Work out the finished part from the listing and answer in its coordinate system (mm). A direction names the side the tool comes from. Give positions to 0.01 mm unless a question says otherwise; leave off trailing zeros. Order: outer loops, then holes, each group sorted by start corner. A loop starts at its lowest first (then second) coordinate and runs counter-clockwise, first axis right, second up. Notation, with made-up numbers: M 30,23 L 83,23 A24 ccw 83,62 Z; hole C 24,-13 d7. An arc over 180 degrees is marked long. One line per item, written item: value.
from build123d import *

# Parameters (mm, degrees)
BOSS_EXTRUDE1_DEPTH  = 5
SKETCH2_R            = 5
CUT_EXTRUDE1_DEPTH   = 5
SKETCH4_W            = 28.341926147
SKETCH4_H            = 5
BOSS_EXTRUDE2_DEPTH  = 5
SKETCH5_W            = 28.341926147
SKETCH5_H            = 5
BOSS_EXTRUDE3_DEPTH  = 31.9
SKETCH6_W            = 20
SKETCH6_H            = 5
CUT_EXTRUDE3_DEPTH   = 5
SKETCH8_W            = 4.170963073
SKETCH8_H            = 5
SKETCH8_W_2          = 4.170963074
BOSS_EXTRUDE8_DEPTH  = 10
SKETCH15_W           = 20
SKETCH15_H           = 5
BOSS_EXTRUDE9_DEPTH  = 5
SKETCH18_W           = 28.341926147
SKETCH18_H           = 5
BOSS_EXTRUDE11_DEPTH = 12.11
SKETCH19_R           = 1
CUT_EXTRUDE6_DEPTH   = 12.11
BOSS_EXTRUDE12_START = 5
SKETCH20_R           = 10
BOSS_EXTRUDE12_DEPTH = 5


with BuildPart() as part:
    # Model → Boss-Extrude1 (new body)
    with BuildSketch(Plane.XY):
        with BuildLine():
            Line((25.203972036, 18.418809181), (53.545898183, 18.418809181))
            ThreePointArc((53.545898183, 18.418809181), (56.325296764, 25.33096224), (62.273132312, 29.817182103))
            ThreePointArc((62.273132312, 29.817182103), (70.250885109, 48.157178295), (51.910888918, 56.134931092))
            ThreePointArc((51.910888918, 56.134931092), (32.934484586, 41.258497646), (25.203972036, 18.418809181))
        make_face()
    extrude(amount=BOSS_EXTRUDE1_DEPTH)

    # Sketch2 → Cut-Extrude1 (cut)
    with BuildSketch(Plane.XY.offset(5)):
        with Locations((57.092010615, 42.976056598)):
            Circle(SKETCH2_R)
    extrude(amount=-CUT_EXTRUDE1_DEPTH, mode=Mode.SUBTRACT)

    # Sketch4 → Boss-Extrude2 (add)
    with BuildSketch(Plane.XZ.offset(-18.418809181)):
        with Locations((39.37493511, 2.5)):
            Rectangle(SKETCH4_W, SKETCH4_H)
    extrude(amount=BOSS_EXTRUDE2_DEPTH)

    # Sketch5 → Boss-Extrude3 (add)
    with BuildSketch(Plane(origin=(0, 0, 0), x_dir=(-1, 0, 0), z_dir=(0, 0, -1))):
        with Locations((-39.37493511, 15.918809181)):
            Rectangle(SKETCH5_W, SKETCH5_H)
    extrude(amount=BOSS_EXTRUDE3_DEPTH)

    # Sketch6 → Cut-Extrude3 (cut)
    with BuildSketch(Plane(origin=(0, 18.418809181, 0), x_dir=(1, 0, 0), z_dir=(0, 1, 0))):
        with Locations((39.37493511, 29.4)):
            Rectangle(SKETCH6_W, SKETCH6_H)
    extrude(amount=-CUT_EXTRUDE3_DEPTH, mode=Mode.SUBTRACT)

    # Sketch8 → Boss-Extrude8 (add)
    with BuildSketch(Plane(origin=(0, 0, -31.9), x_dir=(-1, 0, 0), z_dir=(0, 0, -1))):
        with Locations((-51.460416647, 15.918809181)):
            Rectangle(SKETCH8_W, SKETCH8_H)
        with Locations((-27.289453573, 15.918809181)):
            Rectangle(SKETCH8_W_2, SKETCH8_H)
    extrude(amount=BOSS_EXTRUDE8_DEPTH)

    # Sketch15 → Boss-Extrude9 (add)
    with BuildSketch(Plane(origin=(0, 0, -26.9), x_dir=(-1, 0, 0), z_dir=(0, 0, -1))):
        with Locations((-39.37493511, 15.918809181)):
            Rectangle(SKETCH15_W, SKETCH15_H)
    extrude(amount=BOSS_EXTRUDE9_DEPTH)

    # Sketch18 → Boss-Extrude11 (add)
    with BuildSketch(Plane(origin=(0, 0, -41.9), x_dir=(-1, 0, 0), z_dir=(0, 0, -1))):
        with Locations((-39.37493511, 15.918809181)):
            Rectangle(SKETCH18_W, SKETCH18_H)
    extrude(amount=BOSS_EXTRUDE11_DEPTH)

    # Sketch19 → Cut-Extrude6 (cut)
    with BuildSketch(Plane(origin=(0, 18.418809181, 0), x_dir=(1, 0, 0), z_dir=(0, 1, 0))):
        with Locations(Location((34.37493511, 22, 0), (0, 0, 270))):
            Circle(SKETCH19_R)
        with Locations(Location((44.37493511, 22, 0), (0, 0, 270))):
            Circle(SKETCH19_R)
        with Locations(Location((34.37493511, 15, 0), (0, 0, 270))):
            Circle(SKETCH19_R)
        with Locations(Location((44.37493511, 15, 0), (0, 0, 270))):
            Circle(SKETCH19_R)
    extrude(amount=-CUT_EXTRUDE6_DEPTH, mode=Mode.SUBTRACT)

    # Sketch20 → Boss-Extrude12 (add)
    with BuildSketch(Plane(origin=(0, 0, -54.01), x_dir=(-1, 0, 0), z_dir=(0, 0, -1)).offset(BOSS_EXTRUDE12_START)):
        with BuildLine():
            Line((-53.545898183, 18.418809181), (-53.545898183, 13.418809181))
            Line((-53.545898183, 13.418809181), (-25.203972036, 13.418809181))
            Line((-25.203972036, 13.418809181), (-25.203972036, 18.418809181))
            ThreePointArc((-25.203972036, 18.418809181), (-32.934484586, 41.258497646), (-51.910888918, 56.134931092))
            ThreePointArc((-51.910888918, 56.134931092), (-70.250885109, 48.157178295), (-62.273132312, 29.817182103))
            ThreePointArc((-62.273132312, 29.817182103), (-56.325296764, 25.33096224), (-53.545898183, 18.418809181))
        make_face()
        with Locations((-57.092010615, 42.976056598)):
            Circle(SKETCH20_R, mode=Mode.SUBTRACT)
    extrude(amount=-BOSS_EXTRUDE12_DEPTH)


solid = part.part
(1) Section C-C, the plane y = 40 is taken. Give the vertices of the cut face in (x, z).
Findings:
outline: M 32.08,-59.01 L 47.55,-59.01 L 47.55,-54.01 L 32.08,-54.01 Z; M 32.08,0 L 53.07,0 L 53.07,5 L 32.08,5 Z; M 61.11,0 L 70.92,0 L 70.92,5 L 61.11,5 Z; M 66.64,-59.01 L 70.92,-59.01 L 70.92,-54.01 L 66.64,-54.01 Z
(2) Which of the six approach directions +Z, -Z, +X, -X, +Y, -Y give full straight-line access (tool end or side, diameter ignored) to faces 4 (the flat face through (48, 38, 0)), 5 (the cylindrical face through (52.478, 34.104, -56.545)), 6 (the flat face through (40, 13.419, -27)), 7 (the flat face through (29.375, 16, -37)), 8 (the cylindrical face through (56.261, 25.247, 2.465))?
Findings:
face 4: +X, -X, +Y
face 5: -Z
face 6: +Z, -Z, +X, -X, -Y
face 7: +Y, -Y
face 8: +Z, -Z, +X, -Y
(3) Section A-A, the plane z = -34 is taken. Give the vertices of the cut face in (x, y).
Findings:
outline: M 25.2,13.42 L 29.37,13.42 L 29.37,18.42 L 25.2,18.42 Z; M 49.37,13.42 L 53.55,13.42 L 53.55,18.42 L 49.37,18.42 Z
(4) Section D-D, the plane x = 61 is taken. Give the vertices of the cut face in (y, z).
Findings:
outline: M 29.24,-59.01 L 33.77,-59.01 L 33.77,-54.01 L 29.24,-54.01 Z; M 29.24,0 L 39.86,0 L 39.86,5 L 29.24,5 Z; M 46.09,0 L 56.57,0 L 56.57,5 L 46.09,5 Z; M 52.18,-59.01 L 56.57,-59.01 L 56.57,-54.01 L 52.18,-54.01 Z
(5) Section B-B, the plane z = -22 is taken. Give the vertices of the cut face in (x, y).
Findings:
outline: M 25.2,13.42 L 33.37,13.42 L 33.37,18.42 L 25.2,18.42 Z; M 35.37,13.42 L 43.37,13.42 L 43.37,18.42 L 35.37,18.42 Z; M 45.37,13.42 L 53.55,13.42 L 53.55,18.42 L 45.37,18.42 Z
(6) Determine the mould class of faces 1 (the cylindrical face through (35.218, 15.954, -14.462)), 2 (the cylindrical face through (70.36, 47.87, 2.46)), 3 (the flat face through (43, 31, -59.01)) for opening direction Z: pulls with the +Z half, pulls with the -Z half, needs draft (parallel to the pull), parting line crosses it, or undercut.
Findings:
face 1: undercut
face 2: needs draft
face 3: pulls with the -Z half
(7) Find the intervals of material crossed by probe 1 along X at (y, z) = (16.25, -22); probe 2 along Z at (x, y) = (44.5, 27.5); probe 3 along Z at (x, y) = (59, 49), in increasing order. Write a range as from..to.
Findings:
probe 1: x = 25.2..33.37, 35.37..43.37, 45.37..53.55
probe 2: z = -59.01..-54.01, 0..5
probe 3: z = 0..5
(8) Given P1, Ø1.5, axis at y = 16.5, z = -23.5, coming from the +X side; P2, Ø8.5, axis at x = 39, z = -31, coming from the +Y side; P3, Ø1.2, axis at x = 34.37, z = -15, coming from the -Y side, each flat-ended and moving along its own axis, determine where each tip first touches the part or whether it passes through.
Findings:
P1: stops at x = 53.55
P2: stops at y = 18.42
P3: passes through
